```python
from build123d import *

# Parameters (mm, degrees)
SKETCH_1_R          = 4
EXTRUDE_1_DEPTH     = 12
SKETCH_2_R          = 6
CUT_EXTRUDE_1_DEPTH = 0.2
CUT_EXTRUDE_2_DEPTH = 0.2
SKETCH_5_R          = 0.6
EXTRUDE_2_DEPTH     = 2
SKETCH_7_R          = 2.470632437
CUT_EXTRUDE_3_DEPTH = 0.1
WRAP_START          = 5.798600642
WRAP_1_DEPTH        = 2.284722222
WRAP_START_2        = 8.423600642
WRAP_1_2_DEPTH      = 2.284722222


# Read off the part's stored shape, not the designer's step: 包覆1
with BuildPart() as part:
    # 草图1 → 凸台-拉伸1 (new body)
    with BuildSketch(Plane.XY):
        Circle(SKETCH_1_R)
    extrude(amount=EXTRUDE_1_DEPTH)

    # 草图2 → 切除-拉伸1 (cut)
    with BuildSketch(Plane.XY.offset(12)):
        Circle(SKETCH_2_R)
    extrude(amount=-CUT_EXTRUDE_1_DEPTH, mode=Mode.SUBTRACT)

    # 草图3 → 切除-拉伸2 (cut)
    with BuildSketch(Plane.XY.offset(11.8)):
        with BuildLine():
            Line((-0.04330127, 0.025), (-0.028867513, 0.05))
            Line((-0.028867513, 0.05), (-2.49949995, 0.05))
            ThreePointArc((-2.49949995, 0.05), (-2.5, 0), (-2.49949995, -0.05))
            Line((-2.49949995, -0.05), (-0.028867513, -0.05))
            Line((-0.028867513, -0.05), (-0.04330127, -0.025))
            Line((-0.04330127, -0.025), (0, 0))
            Line((0, 0), (-0.04330127, 0.025))
        make_face()
        with BuildLine():
            Line((0.04330127, -0.025), (0, 0))
            Line((0, 0), (0, -0.05))
            Line((0, -0.05), (-0.028867513, -0.05))
            Line((-0.028867513, -0.05), (1.206448705, -2.189630453))
            ThreePointArc((1.206448705, -2.189630453), (1.25, -2.165063509), (1.293051245, -2.139630453))
            Line((1.293051245, -2.139630453), (0.057735027, 0))
            Line((0.057735027, 0), (0.04330127, -0.025))
        make_face()
        with BuildLine():
            Line((-0.028867513, 0.05), (0, 0.05))
            Line((0, 0.05), (0, 0))
            Line((0, 0), (0.04330127, 0.025))
            Line((0.04330127, 0.025), (0.057735027, 0))
            Line((0.057735027, 0), (1.293051245, 2.139630453))
            ThreePointArc((1.293051245, 2.139630453), (1.25, 2.165063509), (1.206448705, 2.189630453))
            Line((1.206448705, 2.189630453), (-0.028867513, 0.05))
        make_face()
        Polygon((0, 0), (0, 0.05), (-0.028867513, 0.05), (-0.04330127, 0.025), align=None)
        Polygon((0, -0.05), (0, 0), (-0.04330127, -0.025), (-0.028867513, -0.05), align=None)
        Polygon((0.04330127, 0.025), (0, 0), (0.04330127, -0.025), (0.057735027, 0), align=None)
    extrude(amount=-CUT_EXTRUDE_2_DEPTH, mode=Mode.SUBTRACT)

    # 草图4 → 切除-旋转1 (revolve, cut)
    with BuildSketch(Plane(origin=(0, 0, 0), x_dir=(1, 0, 0), z_dir=(0, 1, 0))):
        with BuildLine():
            Line((-4.318421305, -0.940700508), (-4.318421305, -5.059299492))
            ThreePointArc((-4.318421305, -5.059299492), (-3.5, -3), (-4.318421305, -0.940700508))
        make_face()
    revolve(axis=Axis((0, 0, 0), (0, 0, 1)), mode=Mode.SUBTRACT)

    # 草图5 → 凸台-拉伸2 (add)
    with BuildSketch(Plane(origin=(0, 0, 0), x_dir=(-1, 0, 0), z_dir=(0, 0, -1))):
        with Locations(Location((1.5, 0, 0), (0, 0, 180))):
            Circle(SKETCH_5_R)
        with Locations(Location((-1.5, 0, 0), (0, 0, 180))):
            Circle(SKETCH_5_R)
    extrude(amount=EXTRUDE_2_DEPTH)

    # 草图7 → 切除-拉伸3 (cut)
    with BuildSketch(Plane.XY.offset(11.8)):
        with Locations((-0.028867513, -0.05)):
            Circle(SKETCH_7_R)
    extrude(amount=-CUT_EXTRUDE_3_DEPTH, mode=Mode.SUBTRACT)

    # 包覆1 outline → 包覆1 (cut)
    with BuildSketch(Plane.XY.offset(WRAP_START)):
        with BuildLine():
            Line((3.969650484, 0.491807924), (3.77116796, 0.467217528))
            ThreePointArc((3.77116796, 0.467217528), (3.779057907, 0.398398459), (3.785692099, 0.329447005))
            Line((3.785692099, 0.329447005), (3.984939052, 0.346786321))
            ThreePointArc((3.984939052, 0.346786321), (3.977955692, 0.419366799), (3.969650484, 0.491807924))
        make_face()
    extrude(amount=WRAP_1_DEPTH, mode=Mode.SUBTRACT)

    # Wrap 1 2 outline → Wrap 1 2 (cut)
    with BuildSketch(Plane.XY.offset(WRAP_START_2)):
        with BuildLine():
            Line((3.969650484, 0.491807924), (3.77116796, 0.467217528))
            ThreePointArc((3.77116796, 0.467217528), (3.779057907, 0.398398459), (3.785692099, 0.329447005))
            Line((3.785692099, 0.329447005), (3.984939052, 0.346786321))
            ThreePointArc((3.984939052, 0.346786321), (3.977955692, 0.419366799), (3.969650484, 0.491807924))
        make_face()
    extrude(amount=WRAP_1_2_DEPTH, mode=Mode.SUBTRACT)


solid = part.part
```
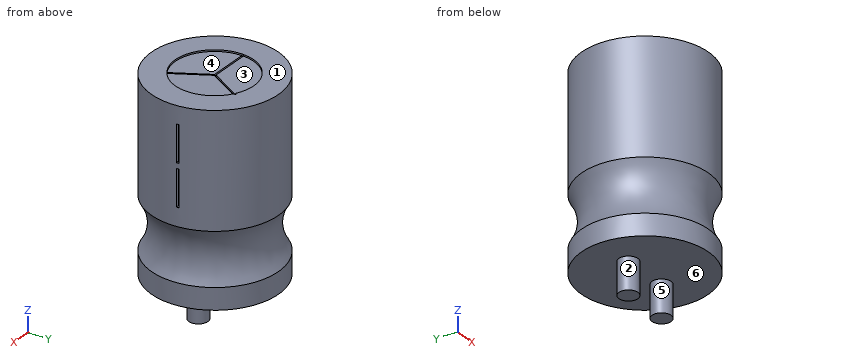
Work out the finished part from the listing and answer in its coordinate system (mm). Face numbers are marked on the shaded views. A direction names the side the tool comes from. Round coordinates to 2 decimals unless told otherwise and drop trailing zeros. Order: outer loops, then holes, each group sorted by start corner. A loop starts at its lowest first (then second) coordinate and runs counter-clockwise, first axis right, second up.
Q1. The mould has two halves that part along Y. Classify the marked faces 4, 5 and 6: pulls with the +Y half, pulls with the -Y half, needs draft (parallel to the pull), parting line crosses it, or undercut.
Solution:
face 4: undercut
face 5: parting line crosses it
face 6: needs draft
Q2. A cutting plane is placed at B-B, the plane z = 5. Determine the outline of the cut face in (x, y), then the cut area to 3 significant figures.
Solution:
outline: circle Ø8 at (0, 0)
area: 50.3 mm2
Q3. A cutting plane is placed at A-A, the plane z = 8.75. Determine the outline of the cut face in (x, y).
Solution:
outline: (3.77, 0.47) - (3.97, 0.49) arc R4 ccw (long way) to (3.98, 0.35) - (3.79, 0.33) arc R3.8 ccw to start
Q4. Given pin 1 Ø3 at (x, y) = (-1, -3) entering from -Z; pin 2 Ø1.2 at (x, y) = (-1.5, 1) entering from +Z; pin 3 Ø3 at (y, z) = (-2, 6.5) entering from +X, each flat-ended and moving along its own axis, determine where each tip first touches the part or whether it passes through.
Solution:
pin 1: stops at z = 0
pin 2: stops at z = 11.7
pin 3: stops at x = 3.97
Q5. A tool of negligible diameter and unlimited length cuts with its end or side. For the marked faces 1, 2 and 3, from which of +Z, -Z, +X, -X, +Y, -Y can it reach the whole face along a straight path? Write none if from no direction.
Solution:
face 1: +Z, +X, -X, +Y, -Y
face 2: -Z
face 3: +Z
Q6. Find the intervals of material crossed by line 1 along Z through (x, y) = (-1.75, -0.25); line 2 along Z through (x, y) = (-2.25, 3); line 3 along Z through (x, y) = (-2.5, -2.25), in increasing order.
Solution:
line 1: z = -2 to 11.7
line 2: z = 0 to 1.8, 4.2 to 11.8
line 3: z = 0 to 11.8
